from build123d import *

# Parameters (mm, degrees)
SKETCH1_R           = 25.4
BOSS_EXTRUDE1_DEPTH = 22.352
SKETCH3_R           = 4.445
CUT_EXTRUDE1_DEPTH  = 12.1760001
CIRPATTERN1_COUNT   = 3
CIRPATTERN1_ANGLE   = 160
SKETCH4_R           = 6.985
SKETCH4_R_2         = 3.683
BOSS_EXTRUDE2_DEPTH = 2.286


with BuildPart() as part:
    # Sketch1 → Boss-Extrude1 (new body)
    with BuildSketch(Plane.XY):
        Circle(SKETCH1_R)
    extrude(amount=BOSS_EXTRUDE1_DEPTH)

    # Sketch2 → Cut-Revolve1 (revolve, cut)
    with BuildSketch(Plane(origin=(0, 0, 11.176), x_dir=(-1, 0, 0), z_dir=(0, 0, -1))):
        with BuildLine():
            Line((0, 25.4), (8.636, 25.4))
            Line((8.636, 25.4), (8.636, 15.748))
            ThreePointArc((8.636, 15.748), (6.106574162, 9.641425838), (0, 7.112))
            Line((0, 7.112), (0, 25.4))
        make_face()
    cut_revolve1 = revolve(axis=Axis((0, 0, 11.176), (0, 1, 0)), mode=Mode.SUBTRACT)

    # Sketch3 → Cut-Extrude1 (cut, symmetric)
    with BuildSketch(Plane(origin=(0, 0, 11.176), x_dir=(-1, 0, 0), z_dir=(0, 0, -1))):
        with Locations((0, 16.256)):
            Circle(SKETCH3_R)
    cut_extrude1 = extrude(amount=CUT_EXTRUDE1_DEPTH, both=True, mode=Mode.SUBTRACT)

    # CirPattern1: Cut-Revolve1, Cut-Extrude1 ×3 about axis
    cirpattern1_axis = Axis((0, 0, 0), (0, 0, -1))
    for i in range(1, CIRPATTERN1_COUNT):
        add(cut_revolve1.rotate(cirpattern1_axis, i * CIRPATTERN1_ANGLE / (CIRPATTERN1_COUNT - 1)), mode=Mode.SUBTRACT)
        add(cut_extrude1.rotate(cirpattern1_axis, i * CIRPATTERN1_ANGLE / (CIRPATTERN1_COUNT - 1)), mode=Mode.SUBTRACT)

    # Sketch4 → Boss-Extrude2 (add)
    with BuildSketch(Plane.XY.offset(22.352)):
        Circle(SKETCH4_R)
        Circle(SKETCH4_R_2, mode=Mode.SUBTRACT)
    extrude(amount=BOSS_EXTRUDE2_DEPTH)


solid = part.part
Work out the finished part from the listing and answer in its coordinate system (mm). A direction names the side the tool comes from. Coordinates: 2 decimals unless noted, no trailing zeros. Loops run counter-clockwise (first coordinate to the right, second up) from the corner with the lowest first, then second, coordinate; pieces in that order, holes last. Notation, with made-up numbers: M 40,45 L 95,45 A26 cw 95,60 Z; hole C 42.25,59.25 d8. An arc over 180 degrees is marked long. Answer in a Markdown table with one row per item. Add a question column.
1. Consider L1, parallel to Z at x = -19, y = 7.5; L2, parallel to Y at x = 2, z = 20; L3, parallel to X at y = 16.5, z = 2. Determine where each line is inside the solid, lowest interval first.
2. Find section C-C, the plane x = -11. Write down the section's boundary in (y, z).
3. The mould has two halves that part along Y. Classify faces 1 (the cylindrical face through (14.754, -16.453, 13.77)), 2 (the flat face through (3, -3, 24.638)), 3 (the cylindrical face through (-0.909, 6.926, 23.479)): pulls with the +Y half, pulls with the -Y half, needs draft (parallel to the pull), parting line crosses it, or undercut.
4. Flat-ended cylindrical pins translate along their axes: P1, Ø11.5, axis at x = 0, y = 16.256, coming from the +Z side; P2, Ø1.5, axis at x = -19.5, z = 12.5, coming from the +Y side; P3, Ø6, axis at x = -15, z = 13, coming from the +Y side. Find the tip coordinate at first contact, or state that the pin passes through.
5. A tool of negligible diameter and unlimited length cuts with its end or side. For faces 4 (the cylindrical face through (3.17, -11.53, 1.86)), 5 (the flat face through (0, 0, 22.352)), 6 (the cylindrical face through (-8.237, 20.507, 13.77)), from which of +Z, -Z, +X, -X, +Y, -Y can it reach the whole face along a straight path? Write none if from no direction.
6. Find section A-A, the plane y = 15. Write down the section's boundary in (x, z).
7. Find section D-D, the plane x = -17. Write down the section's boundary in (y, z).
8. Find section B-B, the plane y = 0. State how many separate pieces and enclosed holes the cut face has, then the cut area to 3 significant figures.
Reported:
| question | item | result |
|---|---|---|
| 1 | L1 | z = 0 to 22.35 |
| 1 | L2 | y = -25.32 to -17.94, -12.61 to 12.29, 20.23 to 25.32 |
| 1 | L3 | x = -19.31 to -4.44, 4.44 to 19.31 |
| 2 | outline | M -22.89,0 L 22.89,0 L 22.89,22.35 L -22.89,22.35 Z |
| 3 | face 1 | undercut |
| 3 | face 2 | needs draft |
| 3 | face 3 | parting line crosses it |
| 4 | P1 | stops at z = 22.35 |
| 4 | P2 | stops at y = 17.13 |
| 4 | P3 | stops at y = 22.39 |
| 5 | face 4 | +Z, -Z |
| 5 | face 5 | +Z |
| 5 | face 6 | +Y |
| 6 | outline | M -20.5,0 L -4.26,0 L -4.26,3.7 A8.6 cw -4.26,18.65 L -4.26,22.35 L -20.5,22.35 Z; M 4.26,0 L 20.5,0 L 20.5,22.35 L 4.26,22.35 L 4.26,18.65 A8.6 cw 4.26,3.7 Z |
| 7 | outline | M -18.87,0 L 18.87,0 L 18.87,22.35 L -18.87,22.35 Z |
| 8 | separate pieces | 3 |
| 8 | enclosed holes | 0 |
| 8 | area | 847 mm^2 |
